Geometry check sheet. Reference: the model listing, model coordinates, mm. Face numbers are marked on the shaded views. A direction names the side the tool comes from. Coordinates: 2 decimals unless noted, no trailing zeros. Write each loop counter-clockwise with the first axis right and the second up, starting at its lowest first coordinate (ties: lowest second). Pieces come first, ordered by that corner, then holes. Notation, with made-up numbers: (60.25, -8) -> (98.25, -8) arc R15 cw to (98.25, 13) -> close; hole circle Ø10 at (-6.75, 86). An arc over 180 degrees is marked (long way). Use a Markdown table: item, result.
Autodesk Fusion 360 part; units mm, degrees
sketch "Cross-section" plane through (0, 0, 0) normal (0, 1, 0) x (1, 0, 0)
  line L0 (0, 0) -> (0, -30) construction
  line L1 (0, 0) -> (21.2132, -21.2132) construction
  arc A0 (0, -30) -> (21.2132, -21.2132) centre (0, 0) ccw
  line L2 (0, -30) -> (-20, -30)
  line L3 (21.2132, -21.2132) -> (35.3553, -7.0711)
  line L4 (19.799, -19.799) -> (33.9411, -5.6569)
  arc A1 (0, -28) -> (19.799, -19.799) centre (0, 0) ccw
  line L5 (0, -28) -> (-20, -28)
  line L6 (-20, -28) -> (-20, -30)
  line L7 (33.9411, -5.6569) -> (35.3553, -7.0711)
  line L8 (0, -29) -> (-15, -29)
  line L9 (21.2132, -21.2132) -> (31.8198, -10.6066)
  dimension "d1" = 60
  dimension "d2" = 45
  dimension "d3" = 20
  dimension "d4" = 20
  dimension "d5" = -2
  dimension "d8" = 15
  dimension "d9" = 15
extrude "Extrude1" add sketch "Cross-section" along normal blind 25
sketch "Mounting_hole_1" plane through (0, 0, 30) normal (0, 0, 1) x (-1, 0, 0)
  line L0 (20, 0) -> (0, 0)
  line L1 (0, 0) -> (0, -25)
  line L2 (0, -25) -> (20, -25)
  line L3 (20, -25) -> (20, 0)
  line L4 (0, -12.5) -> (15, -12.5)
  circle A0 centre (15, -12.5) radius 1.5
  dimension "d10" = 15
  dimension "d11" = 3
extrude "Extrude2" cut sketch "Mounting_hole_1" against normal blind 6 contours A0
sketch "Mounting_hole_2" plane through (21.2132, 0, 21.2132) normal (0.7071, 0, 0.7071) x (0, 1, 0)
  line L0 (0, 0) -> (0, -20)
  line L1 (0, -20) -> (25, -20)
  line L2 (25, -20) -> (25, 0)
  line L3 (25, 0) -> (0, 0)
  line L4 (12.5, 0) -> (12.5, -15)
  circle A0 centre (12.5, -15) radius 1.5
  dimension "d14" = 15
  dimension "d15" = 3
extrude "Extrude3" cut sketch "Mounting_hole_2" against normal blind 8 contours A0
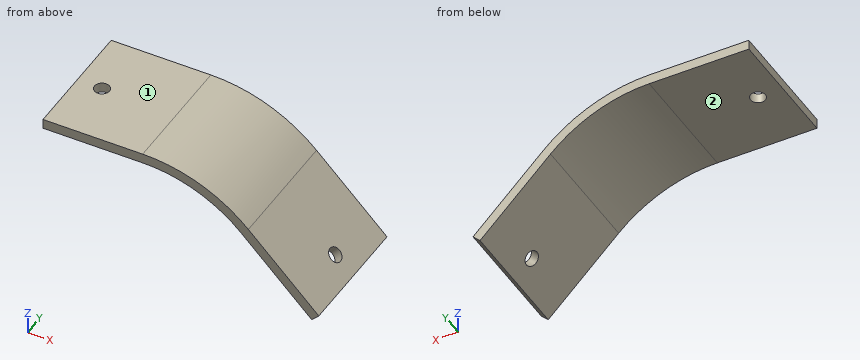
Item 1: Section check A-A on x = -15. Record the boundary of the cut face in (y, z).
Answer block:
| item | result |
|---|---|
| outline | (0, 28) -> (11, 28) -> (11, 30) -> (0, 30) -> close; (14, 28) -> (25, 28) -> (25, 30) -> (14, 30) -> close |
Item 2: Depth check by flat-ended pin: P1, Ø10, axis at y = 12, z = 17, coming from the -X side; P2, Ø12, axis at x = 20.5, z = 22.5, coming from the +Y side; P3, Ø6, axis at x = 9, y = 18.5, coming from the -Z side; P4, Ø3, axis at y = 19.5, z = 9, coming from the +X side. Enter the tip coordinate at first touch or a pass-through.
Answer block:
| item | result |
|---|---|
| P1 | stops at x = 17.32 |
| P2 | stops at y = 25 |
| P3 | stops at z = 25.3 |
| P4 | stops at x = 34.93 |
Item 3: Thickness scan on L1, parallel to Y at x = -15, z = 28.6; L2, parallel to Z at x = -2, y = 6; L3, parallel to X at y = 17.5, z = 6.5. Record the ranges inside material, lowest first. Write a range as [from, to].
Answer block:
| item | result |
|---|---|
| L1 | y = [0, 11], [14, 25] |
| L2 | z = [28, 30] |
| L3 | x = [33.1, 34.78] |
Item 4: Section check C-C on y = 12.5. Record the boundary of the cut face in (x, z), then the cut area to 3 significant figures.
Answer block:
| item | result |
|---|---|
| outline | (-20, 28) -> (-16.5, 28) -> (-16.5, 30) -> (-20, 30) -> close; (-13.5, 28) -> (0, 28) arc R28 cw to (19.8, 19.8) -> (29.34, 10.25) -> (30.76, 11.67) -> (21.21, 21.21) arc R30 ccw to (0, 30) -> (-13.5, 30) -> close; (31.47, 8.13) -> (33.94, 5.66) -> (35.36, 7.07) -> (32.88, 9.55) -> close |
| area | 114 mm^2 |
Item 5: Section check B-B on y = 4. Record the boundary of the cut face in (x, z), then the cut area to 3 significant figures.
Answer block:
| item | result |
|---|---|
| outline | (-20, 28) -> (0, 28) arc R28 cw to (19.8, 19.8) -> (33.94, 5.66) -> (35.36, 7.07) -> (21.21, 21.21) arc R30 ccw to (0, 30) -> (-20, 30) -> close |
| area | 126 mm^2 |
Item 6: Section check D-D on z = 23.75. Record the boundary of the cut face in (x, y).
Answer block:
| item | result |
|---|---|
| outline | (14.83, 0) -> (18.33, 0) -> (18.33, 25) -> (14.83, 25) -> close |
Item 7: Tool access check on the marked faces 1 and 2. Record the directions out of +Z, -Z, +X, -X, +Y, -Y that give a thin tool (end or side, any length) a straight path to the whole face; none if there is none.
Answer block:
| item | result |
|---|---|
| face 1 | +Z, +X, -X, +Y, -Y |
| face 2 | -Z, -X, +Y, -Y |
